Input: part model. Units: mm. Frame: model coordinates. Face numbers are marked on the shaded views. A direction names the side the tool comes from. Coordinates: 2 decimals unless noted, no trailing zeros. Write each loop counter-clockwise with the first axis right and the second up, starting at its lowest first coordinate (ties: lowest second). Pieces come first, ordered by that corner, then holes. Notation, with made-up numbers: M 18,-26.75 L 35,-26.75 A14 ccw 35,-4.75 Z; hole C 84.5,-15.5 d1. An arc over 180 degrees is marked long. Answer as a JSON object with one key per item and string values. Group by question number.
from build123d import *

# Parameters (mm, degrees)
BOSS_EXTRUDE1_DEPTH      = 18.161
BOSS_EXTRUDE1_DEPTH_BACK = 22.3266
SKETCH2_W                = 50.8
SKETCH2_H                = 9.2198
CUT_EXTRUDE1_DEPTH       = 284.270468487
SKETCH3_W                = 16.51
SKETCH3_H                = 3.81
BOSS_EXTRUDE2_DEPTH      = 20.066
FILLET1_R                = 3.175
SKETCH6_R                = 3.5
CUT_EXTRUDE2_DEPTH       = 247.712568685


with BuildPart() as part:
    # Sketch1 → Boss-Extrude1 (new, two sides: drawn at the far end of the back side and taken through both)
    with BuildSketch(Plane(origin=(0, 0, 0), x_dir=(1, 0, 0), z_dir=(0, 1, 0)).offset(-BOSS_EXTRUDE1_DEPTH_BACK)):
        with BuildLine():
            Line((196.889409017, -0.425348601), (198.20116227, 2.041580543))
            ThreePointArc((198.20116227, 2.041580543), (220.828085525, -41.989964588), (187.443785094, -78.544623763))
            Line((187.443785094, -78.544623763), (15.733893811, -93.397170278))
            ThreePointArc((15.733893811, -93.397170278), (4.433186875, -93.703720252), (-6.857314776, -93.134051394))
            ThreePointArc((-6.857314776, -93.134051394), (-93.157259302, -6.53447277), (-19.791883622, 91.264755726))
            Line((-19.791883622, 91.264755726), (-19.791883622, 88.403734249))
            ThreePointArc((-19.791883622, 88.403734249), (-90.355870432, -6.538773964), (-6.857314776, -90.332254043))
            ThreePointArc((-6.857314776, -90.332254043), (4.432766695, -90.912759675), (15.733893811, -90.617036256))
            Line((15.733893811, -90.617036256), (186.839155599, -75.816788928))
            ThreePointArc((186.839155599, -75.816788928), (218.059607792, -41.613105239), (196.889409017, -0.425348601))
        make_face()
    extrude(amount=BOSS_EXTRUDE1_DEPTH + BOSS_EXTRUDE1_DEPTH_BACK)

    # Sketch2 → Cut-Extrude1 (cut, through all)
    with BuildSketch(Plane(origin=(8.135510173, 0, 94.054414573), x_dir=(0.9962799178494617, 0, -0.08617612946674955), z_dir=(0.08617612946674955, 0, 0.9962799178494617))):
        Polygon((131.550880619, -13.1068), (131.550880619, -22.3266), (179.977807149, -22.3266), (179.977807149, -13.1068), (133.582880619, -13.1068), align=None)
        with Locations((205.377807149, -17.7167)):
            Rectangle(SKETCH2_W, SKETCH2_H)
    extrude(amount=-CUT_EXTRUDE1_DEPTH, mode=Mode.SUBTRACT)

    # Sketch3 → Boss-Extrude2 (add)
    with BuildSketch(Plane(origin=(8.135510173, 0, 94.054414573), x_dir=(0.9962799178494617, 0, -0.08617612946674955), z_dir=(0.08617612946674955, 0, 0.9962799178494617))):
        with Locations((123.295880619, -15.0118)):
            Rectangle(SKETCH3_W, SKETCH3_H)
        with Locations((87.735880619, -15.0118)):
            Rectangle(SKETCH3_W, SKETCH3_H)
    extrude(amount=BOSS_EXTRUDE2_DEPTH)

    # Fillet1
    fillet1_edges = [part.edges().sort_by_distance(p)[0] for p in [
        (140.926220923, -15.0118, 102.709221685),
        (124.47763948, -15.0118, 104.131989583),
        (105.498507044, -15.0118, 105.773644849),
        (89.049925601, -15.0118, 107.196412746),
    ]]
    fillet(fillet1_edges, radius=FILLET1_R)

    # Sketch6 → Cut-Extrude2 (cut, through all)
    with BuildSketch(Plane(origin=(0, 0, 0), x_dir=(1, 0, 0), z_dir=(0, 1, 0))):
        with Locations(Location((96.706652463, -98.449712297, 0), (0, 0, 270))):
            Circle(SKETCH6_R)
        with Locations(Location((132.134366342, -95.385289133, 0), (0, 0, 180))):
            Circle(SKETCH6_R)
    extrude(amount=-CUT_EXTRUDE2_DEPTH, mode=Mode.SUBTRACT)


solid = part.part
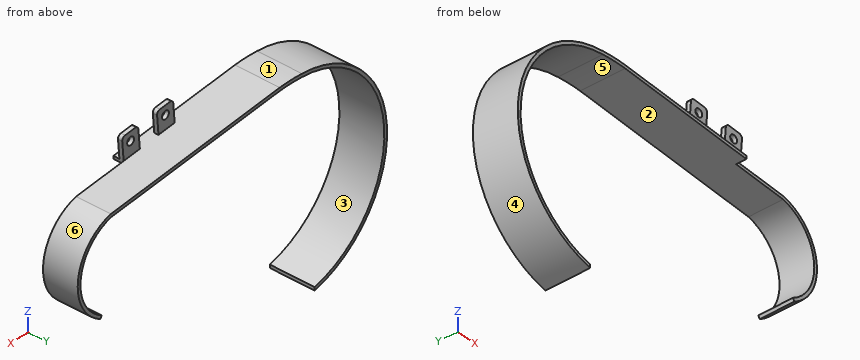
Q1. Pin query (flat end, axial travel): pin 1 Ø9 at (x, z) = (96, 99) entering from +Y; pin 2 Ø5 at (y, z) = (-3.5, -6.5) entering from +X; pin 3 Ø1.4 at (y, z) = (3, -89.5) entering from +X. Return the tip coordinate at first contact, or that it passes through.
Q2. Section A-A, the plane z = 28.5. Return the cut outline in (x, y).
Q3. Access query for the marked faces 1, 2 and 3. Directions: +Z, -Z, +X, -X, +Y, -Y. A direction counts if a zero-diameter tool reaches every point of the face in a straight line with its end or side. Return the directions, or none.
Q4. Section C-C, the plane z = 8.5. Return the cut outline in (x, y), and give its area (3 significant figures).
Q5. Section D-D, the plane x = 7.5. Return the cut outline in (y, z).
Q6. Section B-B, the plane y = 9. Return the cut outline in (x, z), and give its area (3 significant figures).
Q7. Line query: line 1 (Z direction, x = -41, y = -18); line 2 (X direction, y = 8, z = 63); line 3 (Z direction, x = -76.5, y = 5). Output: solid intervals per line, ascending. Write a range as from..to.
Q8. Draft query along X for the marked faces 4, 5 and 6. Return one class per face: released by +X, released by -X, zero draft, split by the parting line, or undercut.
Filled in:
{
 "1": {"pin 1": "y = -13.11", "pin 2": "x = -90.14", "pin 3": "x = -19.79"},
 "2": {"outline": "M -88.93,-22.33 L -85.99,-22.33 L -85.99,18.16 L -88.93,18.16 Z; M 217.67,-13.11 L 220.51,-13.11 L 220.51,18.16 L 217.67,18.16 Z"},
 "3": {"face 1": "+Z, +Y, -Y", "face 2": "-Z, +Y, -Y", "face 3": "+Y, -Y"},
 "4": {"outline": "M -93,-22.33 L -90.19,-22.33 L -90.19,18.16 L -93,18.16 Z; M 207.44,-13.11 L 211.17,-13.11 L 211.17,18.16 L 207.44,18.16 Z", "area": "230 mm^2"},
 "5": {"outline": "M -22.33,90.92 L 18.16,90.92 L 18.16,93.71 L -22.33,93.71 Z"},
 "6": {"outline": "M -19.79,-91.26 L -19.79,-88.4 A90.59 cw -6.86,90.33 A145.84 cw 15.73,90.62 L 186.84,75.82 A40.58 cw 196.89,0.43 L 198.2,-2.04 A43.37 ccw 187.44,78.54 L 15.73,93.4 A145.84 ccw -6.86,93.13 A93.39 ccw Z", "area": "1,560 mm^2"},
 "7": {"line 1": "-83.9..-80.78, 80.78..83.9", "line 2": "-68.93..-65.1, 208.35..211.98", "line 3": "-53.56..-48.53, 48.53..53.56"},
 "8": {"face 4": "released by -X", "face 5": "undercut", "face 6": "released by +X"}
}
